Geometry: final body of the model. Coordinates: model frame, mm. Face numbers are marked on the shaded views. A direction names the side the tool comes from. Round coordinates to 2 decimals unless told otherwise and drop trailing zeros. Order: outer loops, then holes, each group sorted by start corner. A loop starts at its lowest first (then second) coordinate and runs counter-clockwise, first axis right, second up. Notation, with made-up numbers: (-9.75, 46.25) -> (40.25, 46.25) arc R17 ccw to (40.25, 56.25) -> close; hole circle Ø9 at (-17.75, 39.25). An arc over 180 degrees is marked (long way). Put each result on its own line as item: value.
```python
from build123d import *

# Parameters (mm, degrees)
F2_DEPTH      = 38.1
F4_DEPTH      = 12.7
F4_DEPTH_BACK = 96.52
F5_R          = 5.08
F7_R          = 5.08
F8_R          = 5.08


with BuildPart() as f2:
    # F1 (on Top) → F2 (new body)
    with BuildSketch(Plane.XY):
        Polygon((-25.4, 27.94), (-44.45, 0), (44.45, 0), (25.4, 27.94), align=None)
        Polygon((-37.240951, 3.81), (-23.386406, 24.13), (23.386406, 24.13), (37.240951, 3.81), align=None, mode=Mode.SUBTRACT)
        Polygon((23.386406, 24.13), (-23.386406, 24.13), (-37.240951, 3.81), (37.240951, 3.81), align=None)
    extrude(amount=F2_DEPTH)

    # F3 (on offset) → F4 (join, two sides)
    with BuildSketch(Plane.YZ.offset(41.91)) as f4_sk:
        with BuildLine():
            ThreePointArc((-3.437933, -10.16), (3.84106, 4.050015), (6.35, 19.817498))
            ThreePointArc((6.35, 19.817498), (4.124015, 34.690461), (-2.35886, 48.26))
            Line((-2.35886, 48.26), (-5.46216, 48.26))
            ThreePointArc((-5.46216, 48.26), (1.433443, 34.775346), (3.81, 19.817498))
            ThreePointArc((3.81, 19.817498), (1.125414, 3.945848), (-6.629672, -10.16))
            Line((-6.629672, -10.16), (-3.437933, -10.16))
        make_face()
        with BuildLine():
            ThreePointArc((3.81, 19.817498), (1.433443, 34.775346), (-5.46216, 48.26))
            Line((-5.46216, 48.26), (-6.629672, -10.16))
            ThreePointArc((-6.629672, -10.16), (1.125414, 3.945848), (3.81, 19.817498))
        make_face()
    extrude(amount=F4_DEPTH)
    extrude(f4_sk.sketch, amount=-F4_DEPTH_BACK)

    # F5
    f5_edges = [f2.edges().sort_by_distance(p)[0] for p in [
        (25.4, 27.94, 19.05),
        (-25.4, 27.94, 19.05),
    ]]
    fillet(f5_edges, radius=F5_R)

    # F7
    f7_edges = [f2.edges().sort_by_distance(p)[0] for p in [
        (34.888585, 14.023408, 0),
    ]]
    fillet(f7_edges, radius=F7_R)

    # F8
    f8_edges = [f2.edges().sort_by_distance(p)[0] for p in [
        (-34.67687, 14.333925, 38.1),
    ]]
    fillet(f8_edges, radius=F8_R)


solid = f2.part
```
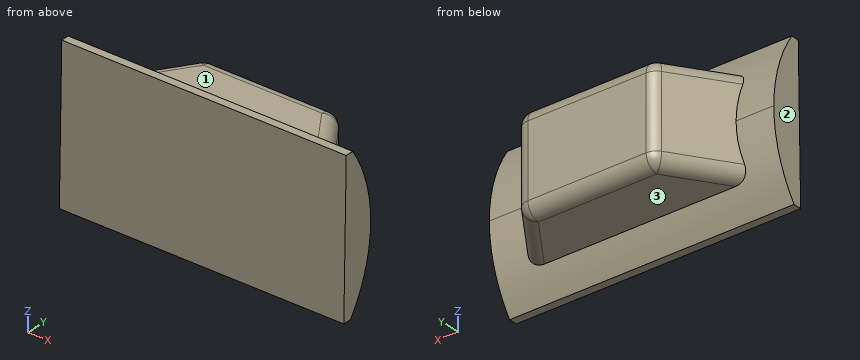
1. Cut plane C-C on x = 16. Return loops of the section in (y, z).
Ans:
outline: (-6.63, -10.16) -> (-3.44, -10.16) arc R50.8 ccw to (2.33, 0) -> (22.86, 0) arc R5.08 ccw to (27.94, 5.08) -> (27.94, 33.02) arc R5.08 ccw to (22.86, 38.1) -> (2.95, 38.1) arc R50.8 ccw to (-2.36, 48.26) -> (-5.46, 48.26) -> close
2. Material intervals for probe 1 along Z at (x, y) = (-25, 8.5); probe 2 along Y at (x, z) = (-1, 5.5); probe 3 along Y at (x, z) = (-6, 13.5), sorted ascending.
Ans:
probe 1: 0 to 38.1
probe 2: -6.32 to 27.94
probe 3: -6.16 to 27.94
3. Set-up query: the marked faces 1, 2 and 3. Return all of +Z, -Z, +X, -X, +Y, -Y with unobstructed straight access to the full face (end or side cutting, diameter ignored); none if empty.
Ans:
face 1: +Z, +X, -X, +Y
face 2: +Z, -Z, -X, +Y, -Y
face 3: -Z, +X, -X, +Y
4. Cut plane D-D on y = 1. Return loops of the section in (x, z), and give its area (3 significant figures).
Ans:
outline: (-54.61, -2.87) -> (54.61, -2.87) -> (54.61, 42.51) -> (-54.61, 42.51) -> close
area: 4,960 mm²
5. Cut plane B-B on z = 23. Return loops of the section in (x, y).
Ans:
outline: (-54.61, -5.97) -> (54.61, -5.97) -> (54.61, 6.25) -> (40.19, 6.25) -> (26.91, 25.72) arc R5.08 ccw to (22.72, 27.94) -> (-22.72, 27.94) arc R5.08 ccw to (-26.91, 25.72) -> (-40.19, 6.25) -> (-54.61, 6.25) -> close
6. Contact query for flat-ended pins moving along their axis: P1, Ø8, axis at x = 21.5, z = -2, coming from the -Y side; P2, Ø10, axis at x = 9.5, y = 8.5, coming from the +Z side; P3, Ø10, axis at x = -32.5, z = 11.5, coming from the +Y side. Output: stop coordinate, or through.
Ans:
P1: y = -6.55
P2: z = 38.1
P3: y = 24.86
7. Cut plane A-A on x = -46.5. Return loops of the section in (y, z), and give its area (3 significant figures).
Ans:
outline: (-6.63, -10.16) -> (-3.44, -10.16) arc R50.8 ccw to (6.35, 19.82) arc R50.8 ccw to (-2.36, 48.26) -> (-5.46, 48.26) -> close
area: 551 mm²
